```python
from build123d import *

# Parameters (mm, degrees)
BOSS_EXTRUDE1_DEPTH = 8
SKETCH7_R           = 1.6
CUT_EXTRUDE2_DEPTH  = 8
SKETCH12_R          = 1.25
CUT_EXTRUDE6_DEPTH  = 10
SKETCH13_R          = 2.9
CUT_EXTRUDE7_DEPTH  = 4
SKETCH14_R          = 2.3
CUT_EXTRUDE8_DEPTH  = 3


with BuildPart() as part:
    # Sketch4 → Boss-Extrude1 (new body)
    with BuildSketch(Plane.XY):
        with BuildLine():
            Line((-26.462284272, 148.586666667), (-18.473670152, -0.986666667))
            ThreePointArc((-18.473670152, -0.986666667), (0, -18.5), (18.473670152, -0.986666667))
            Line((18.473670152, -0.986666667), (26.462284272, 148.586666667))
            ThreePointArc((26.462284272, 148.586666667), (21.489637404, 165.506304662), (7, 175.558755838))
            Line((7, 175.558755838), (7, 169.267848868))
            ThreePointArc((7, 169.267848868), (0, 129.5), (-7, 169.267848868))
            Line((-7, 169.267848868), (-7, 175.558755838))
            ThreePointArc((-7, 175.558755838), (-21.489637404, 165.506304662), (-26.462284272, 148.586666667))
        make_face()
    extrude(amount=BOSS_EXTRUDE1_DEPTH)

    # Sketch7 → Cut-Extrude2 (cut)
    with BuildSketch(Plane.XY.offset(8)):
        with Locations((0, -13.5)):
            Circle(SKETCH7_R)
        with Locations((-11.691342951, 6.75)):
            Circle(SKETCH7_R)
        with Locations((11.691342951, 6.75)):
            Circle(SKETCH7_R)
    extrude(amount=-CUT_EXTRUDE2_DEPTH, mode=Mode.SUBTRACT)

    # Sketch12 → Cut-Extrude6 (cut)
    with BuildSketch(Plane.XY.offset(8)):
        with Locations((23.75, 150)):
            Circle(SKETCH12_R)
        with Locations((11.875, 129.43189666)):
            Circle(SKETCH12_R)
        with Locations((-11.875, 129.43189666)):
            Circle(SKETCH12_R)
        with Locations((-23.75, 150)):
            Circle(SKETCH12_R)
        with Locations((-11.875, 170.56810334)):
            Circle(SKETCH12_R)
        with Locations((11.875, 170.56810334)):
            Circle(SKETCH12_R)
    extrude(amount=-CUT_EXTRUDE6_DEPTH, mode=Mode.SUBTRACT)

    # Sketch13 → Cut-Extrude7 (cut)
    with BuildSketch(Plane.XY.offset(8)):
        with Locations((-11.691342951, 6.75)):
            Circle(SKETCH13_R)
        with Locations((11.691342951, 6.75)):
            Circle(SKETCH13_R)
        with Locations((0, -13.5)):
            Circle(SKETCH13_R)
    extrude(amount=-CUT_EXTRUDE7_DEPTH, mode=Mode.SUBTRACT)

    # Sketch14 → Cut-Extrude8 (cut)
    with BuildSketch(Plane.XY.offset(8)):
        with Locations((23.75, 150)):
            Circle(SKETCH14_R)
        with Locations((11.875, 129.43189666)):
            Circle(SKETCH14_R)
        with Locations((-11.875, 129.43189666)):
            Circle(SKETCH14_R)
        with Locations((-23.75, 150)):
            Circle(SKETCH14_R)
        with Locations((-11.875, 170.56810334)):
            Circle(SKETCH14_R)
        with Locations((11.875, 170.56810334)):
            Circle(SKETCH14_R)
    extrude(amount=-CUT_EXTRUDE8_DEPTH, mode=Mode.SUBTRACT)


solid = part.part
```
Source: CAD feature listing. Evaluate the final solid. Frame: model axes, mm. A direction names the side the tool comes from. Round coordinates to 2 decimals unless told otherwise and drop trailing zeros. Loops run counter-clockwise (first coordinate to the right, second up) from the corner with the lowest first, then second, coordinate; pieces in that order, holes last. Notation, with made-up numbers: (86.25, 67.5) - (107.25, 67.5) arc R19 cw to (107.25, 102.5) - close; hole circle Ø2 at (-36, -19.75). An arc over 180 degrees is marked (long way). Use CSV: the item, a comma, the result in double quotes.
Q1. Section query D-D, the plane x = 5. Output: boundary loops of the cut face in (y, z), then the cut area to 3 significant figures.
Reported:
outline,"(-17.81, 0) - (130.12, 0) - (130.12, 8) - (-17.81, 8) - close"
area,"1,180 mm^2"
Q2. Mould query, pull axis X, two halves, no side actions, for faces 4 (the cylindrical face through (21.636, 165.302, 3.944)), 5 (the flat face through (-22.524, 74.847, 3.944)), 6 (the flat face through (0, 80, 0)), 7 (the cylindrical face through (-22.514, 151.939, 6.521)). Classes: pulls with the +X half, pulls with the -X half, needs draft (parallel to the pull), parting line crosses it, or undercut.
Reported:
face 4,"pulls with the +X half"
face 5,"pulls with the -X half"
face 6,"needs draft"
face 7,"undercut"
Q3. Ray query, line 1 along X through (y, z) = (149, 7.25); line 2 along Z through (x, y) = (-12.5, 168.5); line 3 along Y through (x, z) = (1, 3.75). Return the intervals inside material, ascending.
Reported:
line 1,"-26.48 to -25.82, -21.68 to -20.48, 20.48 to 21.68, 25.82 to 26.48"
line 2,"0 to 5"
line 3,"-18.47 to -14.75, -12.25 to 129.52"
Q4. Pin query (flat end, axial travel): pin 1 Ø3 at (y, z) = (55, 2) entering from +X; pin 2 Ø4 at (x, y) = (-11.88, 129.43) entering from +Z; pin 3 Ø4 at (y, z) = (42.5, 7) entering from +X; pin 4 Ø2 at (x, y) = (11.88, 170.57) entering from -Z. Return the tip coordinate at first contact, or that it passes through.
Reported:
pin 1,"x = 21.54"
pin 2,"z = 5"
pin 3,"x = 20.9"
pin 4,"through"
Q5. Reachability of faces 1 (the cylindrical face through (11.576, 131.712, 6.521)), 2 (the flat face through (0, 80, 8)), 3 (the flat face through (-7, 172, 4)) from +Z, -Z, +X, -X, +Y, -Y: full face, straight path, thin tool, end or side. Return the list, or none.
Reported:
face 1,"+Z"
face 2,"+Z, +X, -X, +Y, -Y"
face 3,"+Z, -Z, +Y"
Q6. Section query A-A, the plane x = -16.5. Output: boundary loops of the cut face in (y, z).
Reported:
outline,"(-8.37, 0) - (137.83, 0) - (137.83, 8) - (-8.37, 8) - close; (162.17, 0) - (170.74, 0) - (170.74, 8) - (162.17, 8) - close"
Q7. Section query C-C, the plane y = 104.5. Output: boundary loops of the cut face in (x, z).
Reported:
outline,"(-24.11, 0) - (24.11, 0) - (24.11, 8) - (-24.11, 8) - close"
Q8. Section query B-B, the plane z = 1.25. Give the number of separate pieces and of enclosed holes in the cut face, then the cut area to 3 significant figures.
Reported:
separate pieces,"1"
enclosed holes,"9"
area,"6,940 mm^2"
